The listing builds one solid part. Answer for the finished solid, in the listing's coordinates (mm). A direction names the side the tool comes from. Coordinates: 2 decimals unless noted, no trailing zeros. Write each loop counter-clockwise with the first axis right and the second up, starting at its lowest first coordinate (ties: lowest second). Pieces come first, ordered by that corner, then holes.
from build123d import *

# Parameters (mm, degrees)
SKETCH_1_R      = 1.5
SKETCH_1_W      = 5.2
SKETCH_1_H      = 2.2
EXTRUDE_1_DEPTH = 2


with BuildPart() as part:
    # 草图1 → 凸台-拉伸1 (new body)
    with BuildSketch(Plane.XY):
        with BuildLine():
            Line((-11, 0), (-11, -3))
            Line((-11, -3), (11, -3))
            Line((11, -3), (11, 0))
            Line((11, 0), (11, 3))
            Line((11, 3), (4.4, 3))
            Line((4.4, 3), (4.4, 73))
            Line((4.4, 73), (0.486767159, 97.013019707))
            Line((0.486767159, 97.013019707), (0, 97.013019707))
            Line((0, 97.013019707), (0, 95.013019707))
            Line((0, 95.013019707), (-4.4, 73))
            ThreePointArc((-4.4, 73), (-1.88316536, 70.48316536), (-4.4, 67.966330721))
            Line((-4.4, 67.966330721), (-4.4, 53.848593982))
            ThreePointArc((-4.4, 53.848593982), (-2.002653764, 51.451247746), (-4.4, 49.053901511))
            Line((-4.4, 49.053901511), (-4.4, 38))
            ThreePointArc((-4.4, 38), (-1.912982257, 35.512982257), (-4.4, 33.025964514))
            Line((-4.4, 33.025964514), (-4.4, 15.982889536))
            ThreePointArc((-4.4, 15.982889536), (-1.348558079, 12.931447615), (-4.4, 9.880005694))
            Line((-4.4, 9.880005694), (-4.4, 3))
            Line((-4.4, 3), (-11, 3))
            Line((-11, 3), (-11, 0))
        make_face()
        Circle(SKETCH_1_R, mode=Mode.SUBTRACT)
        with Locations((7, 0)):
            Rectangle(SKETCH_1_W, SKETCH_1_H, mode=Mode.SUBTRACT)
        with Locations((-7, 0)):
            Rectangle(SKETCH_1_W, SKETCH_1_H, mode=Mode.SUBTRACT)
    extrude(amount=EXTRUDE_1_DEPTH)


solid = part.part
1. Section B-B on y = 0 is taken. Give the vertices of the cut face in (x, z).
Results found:
outline: (-11, 0) - (-9.6, 0) - (-9.6, 2) - (-11, 2) - close; (-4.4, 0) - (-1.5, 0) - (-1.5, 2) - (-4.4, 2) - close; (1.5, 0) - (4.4, 0) - (4.4, 2) - (1.5, 2) - close; (9.6, 0) - (11, 0) - (11, 2) - (9.6, 2) - close
2. Section C-C on x = 8.75 is taken. Give the vertices of the cut face in (y, z).
Results found:
outline: (-3, 0) - (-1.1, 0) - (-1.1, 2) - (-3, 2) - close; (1.1, 0) - (3, 0) - (3, 2) - (1.1, 2) - close
3. Flat-ended cylindrical pins translate along their axes: P1, Ø1, axis at y = 45, z = 1, coming from the -X side; P2, Ø12, axis at x = 0.5, y = 77, coming from the -Z side; P3, Ø1, axis at y = 96, z = 1.5, coming from the -X side; P4, Ø0.6, axis at x = -7.5, z = 1, coming from the +Y side. Find the tip coordinate at first contact, or state that the pin passes through.
Results found:
P1: stops at x = -4.4
P2: stops at z = 0
P3: stops at x = 0
P4: stops at y = 3
4. A tool of negligible diameter and unlimited length cuts with its end or side. For faces 1 (the flat face through (7, 1.1, 1)), 2 (the flat face through (-4.4, 6, 1)), 3 (the cylindrical face through (-1.914, 35.568, 0.986)), 4 (the flat face through (4.4, 38, 1)), from which of +Z, -Z, +X, -X, +Y, -Y can it reach the whole face along a straight path? Write none if from no direction.
Results found:
face 1: +Z, -Z
face 2: +Z, -Z, -X, +Y
face 3: +Z, -Z, -X
face 4: +Z, -Z, +X, +Y
5. Find the intervals of material crossed by L1, parallel to Y at x = -7, z = 0.55; L2, parallel to X at y = 54, z = 0.75; L3, parallel to X at y = 51.5, z = 0.4, in increasing order.
Results found:
L1: y = -3 to -1.1, 1.1 to 3
L2: x = -4.4 to 4.4
L3: x = -2 to 4.4
6. Section D-D on x = -3.5 is taken. Give the vertices of the cut face in (y, z).
Results found:
outline: (-3, 0) - (10.02, 0) - (10.02, 2) - (-3, 2) - close; (15.85, 0) - (33.19, 0) - (33.19, 2) - (15.85, 2) - close; (37.83, 0) - (49.23, 0) - (49.23, 2) - (37.83, 2) - close; (53.67, 0) - (68.13, 0) - (68.13, 2) - (53.67, 2) - close; (72.83, 0) - (77.5, 0) - (77.5, 2) - (72.83, 2) - close
7. For a pull along X with two mould halves and no side action, classify faces 5 (the flat face through (-2.17, 84.16, 0.99)), 6 (the flat face through (-4.4, 0, 1)), 7 (the flat face through (1, 36, 2)), 8 (the flat face through (11, 0, 1)) as pulls with the +X half, pulls with the -X half, needs draft (parallel to the pull), parting line crosses it, or undercut.
Results found:
face 5: pulls with the -X half
face 6: undercut
face 7: needs draft
face 8: pulls with the +X half
8. Section A-A on z = 1.35 is taken. Give the vertices of the cut face in (x, y).
Results found:
outline: (-11, -3) - (11, -3) - (11, 3) - (4.4, 3) - (4.4, 73) - (0.49, 97.01) - (0, 97.01) - (0, 95.01) - (-4.4, 73) arc R2.52 cw to (-4.4, 67.97) - (-4.4, 53.85) arc R2.4 cw to (-4.4, 49.05) - (-4.4, 38) arc R2.49 cw to (-4.4, 33.03) - (-4.4, 15.98) arc R3.05 cw to (-4.4, 9.88) - (-4.4, 3) - (-11, 3) - close; hole (-9.6, -1.1) - (-4.4, -1.1) - (-4.4, 1.1) - (-9.6, 1.1) - close; hole circle Ø3 at (0, 0); hole (4.4, -1.1) - (9.6, -1.1) - (9.6, 1.1) - (4.4, 1.1) - close
